Part model, mm, in its own coordinate system. Give positions to 0.01 mm unless a question says otherwise; leave off trailing zeros. Write each loop counter-clockwise with the first axis right and the second up, starting at its lowest first coordinate (ties: lowest second). Pieces come first, ordered by that corner, then holes. Notation, with made-up numbers: M 5.5,29 L 20.5,29 A6 ccw 20.5,36 Z; hole C -38,23.5 d4. An arc over 180 degrees is marked long. Use a Markdown table: item, result.
```python
from build123d import *

# Parameters (mm, degrees)
F0_R     = 3.75
F1_DEPTH = 3


with BuildPart() as f1:
    # F0 (on Front) → F1 (new body)
    with BuildSketch(Plane.XZ):
        with BuildLine():
            ThreePointArc((15.103494, -0.10421), (4.430052, -4.460724), (0, -15.103853))
            Line((0, -15.103853), (0, -65))
            ThreePointArc((0, -65), (4.393398, -75.606602), (15, -80))
            Line((15, -80), (110, -80))
            ThreePointArc((110, -80), (120.606602, -84.393398), (125, -95))
            Line((125, -95), (125, -195))
            ThreePointArc((125, -195), (129.393398, -205.606602), (140, -210))
            Line((140, -210), (213.46438, -210))
            ThreePointArc((213.46438, -210), (224.574304, -205.078174), (228.393413, -193.542612))
            Line((228.393413, -193.542612), (214.319188, -49.370563))
            ThreePointArc((214.319188, -49.370563), (209.468329, -39.718027), (199.390155, -35.82795))
            Line((199.390155, -35.82795), (119.997144, -35.82795))
            Line((119.997144, -35.82795), (119.997144, -15.724811))
            ThreePointArc((119.997144, -15.724811), (115.640273, -5.154863), (105.100638, -0.725168))
            Line((105.100638, -0.725168), (15.103494, -0.10421))
        make_face()
        with Locations((138, -197)):
            Circle(F0_R, mode=Mode.SUBTRACT)
        with Locations((138, -132)):
            Circle(F0_R, mode=Mode.SUBTRACT)
        with Locations((13, -67)):
            Circle(F0_R, mode=Mode.SUBTRACT)
        with Locations((62.5, -67)):
            Circle(F0_R, mode=Mode.SUBTRACT)
        with Locations((13, -13.090006)):
            Circle(F0_R, mode=Mode.SUBTRACT)
        with Locations((106.997144, -13.738563)):
            Circle(F0_R, mode=Mode.SUBTRACT)
        with Locations((138, -67)):
            Circle(F0_R, mode=Mode.SUBTRACT)
    extrude(amount=F1_DEPTH)


solid = f1.part
```
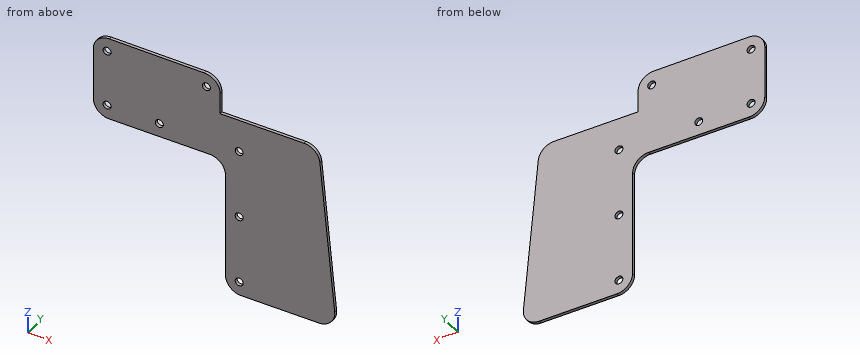
1. Cut at C-C, the plane x = 62.5. Give the cut face in (y, z).
Findings below:
| item | result |
|---|---|
| outline | M -3,-80 L 0,-80 L 0,-70.75 L -3,-70.75 Z; M -3,-63.25 L 0,-63.25 L 0,-0.43 L -3,-0.43 Z |
2. Drop flat-ended pins along their axis: P1, Ø0.9, axis at y = -1.5, z = -121.5, coming from the -X side; P2, Ø1.5, axis at x = 67.5, y = -2, coming from the -Z side; P3, Ø0.9, axis at x = 141.5, y = -1.5, coming from the +Z side. Give the stop position or say it passes through.
Findings below:
| item | result |
|---|---|
| P1 | x = 125 |
| P2 | z = -80 |
| P3 | z = -35.83 |
3. Cut at D-D, the plane x = 195. Give the cut face in (y, z).
Findings below:
| item | result |
|---|---|
| outline | M -3,-210 L 0,-210 L 0,-35.83 L -3,-35.83 Z |
4. Drill centre lines: L1, parallel to Z at x = 13, y = -2.4; L2, parallel to X at y = -1.25, z = -32; L3, parallel to X at y = -2.7, z = -69.5. Where is each one in solid material? Low to high.
Findings below:
| item | result |
|---|---|
| L1 | -79.87 to -70.75, -63.25 to -16.84, -9.34 to -0.24 |
| L2 | 0 to 120 |
| L3 | 0.69 to 10.2, 15.8 to 59.7, 65.3 to 135.2, 140.8 to 216.28 |
5. Cut at A-A, the plane z = -132. Give the cut face in (x, y).
Findings below:
| item | result |
|---|---|
| outline | M 125,-3 L 134.25,-3 L 134.25,0 L 125,0 Z; M 141.75,-3 L 222.39,-3 L 222.39,0 L 141.75,0 Z |
6. Cut at B-B, the plane y = -0.5. Give the cut face in (x, z).
Findings below:
| item | result |
|---|---|
| outline | M 0,-65 A15 ccw 15,-80 L 110,-80 A15 cw 125,-95 L 125,-195 A15 ccw 140,-210 L 213.46,-210 A15 ccw 228.39,-193.54 L 214.32,-49.37 A15 ccw 199.39,-35.83 L 120,-35.83 L 120,-15.72 A15 ccw 105.1,-0.73 L 15.1,-0.1 A15 ccw 0,-15.1 Z; hole C 13,-67 d7.5; hole C 13,-13.09 d7.5; hole C 62.5,-67 d7.5; hole C 107,-13.74 d7.5; hole C 138,-197 d7.5; hole C 138,-132 d7.5; hole C 138,-67 d7.5 |
